Read the model definition and answer for the solid it produces. Units are mm, in the model's axes. Face numbers are marked on the shaded views. A direction names the side the tool comes from. Coordinates: 2 decimals unless noted, no trailing zeros. Write each loop counter-clockwise with the first axis right and the second up, starting at its lowest first coordinate (ties: lowest second). Pieces come first, ordered by that corner, then holes. Notation, with made-up numbers: (-25.5, 87.25) -> (-4.5, 87.25) arc R17 ccw to (-4.5, 113.25) -> close; hole circle Ø6 at (-38, 11.5). An arc over 180 degrees is marked (long way). Return JSON: item names as keys, results as strings.
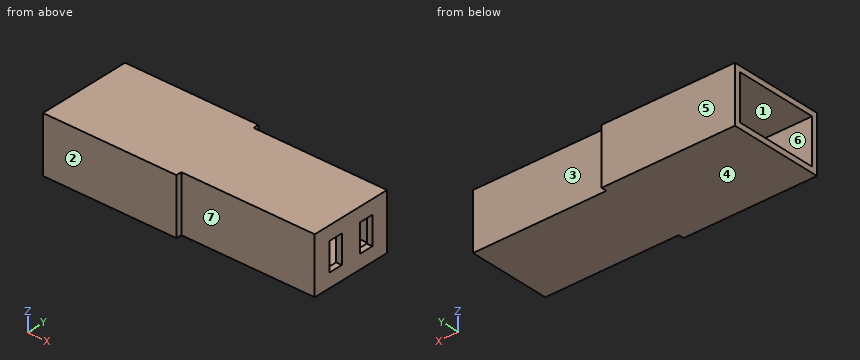
from build123d import *

# Parameters (mm, degrees)
F1_DEPTH = 4
F2_T     = -0.4
F3_W     = 1
F3_H     = 2
F4_DEPTH = 0.4


with BuildPart() as f1:
    # F0 (on Top) → F1 (new body)
    with BuildSketch(Plane.XY):
        Polygon((0, 3.35), (0, -3.35), (9.5, -3.35), (9.5, -2.95), (19, -2.95), (19, 2.95), (9.5, 2.95), (9.5, 3.35), align=None)
    extrude(amount=F1_DEPTH)

    # F2
    f2_openings = [f1.faces().sort_by_distance(p)[0] for p in [
        (0, 0, 2),
    ]]
    offset(amount=F2_T, openings=f2_openings, kind=Kind.INTERSECTION)

    # F3 (on face) → F4 (cut, through all)
    with BuildSketch(Plane.YZ.offset(19)):
        with Locations((-1.2436551969, 2)):
            Rectangle(F3_W, F3_H)
        with Locations((1.2563448031, 2)):
            Rectangle(F3_W, F3_H)
    extrude(amount=-F4_DEPTH, mode=Mode.SUBTRACT)


solid = f1.part
1. A tool of negligible diameter and unlimited length cuts with its end or side. For the marked faces 5, 6 and 7, from which of +Z, -Z, +X, -X, +Y, -Y can it reach the whole face along a straight path? Write none if from no direction.
Taken from the geometry:
{"face 5": "+Z, -Z, +X, -X, +Y", "face 6": "-X", "face 7": "+Z, -Z, +X, -Y"}
2. For a pull along Y with two mould halves and no side action, classify the marked faces 1, 2, 3 and 4 as +Y half, -Y half, draft (parallel to the pull), parting line (faces both ways), or undercut.
Taken from the geometry:
{"face 1": "undercut", "face 2": "-Y half", "face 3": "+Y half", "face 4": "draft"}
3. The part is cut by section C-C (z = 1.95). Determine the outline of the cut face in (x, y), then the cut area to 3 significant figures.
Taken from the geometry:
{"outline": "(0, -3.35) -> (9.5, -3.35) -> (9.5, -2.95) -> (19, -2.95) -> (19, -1.74) -> (18.6, -1.74) -> (18.6, -2.55) -> (9.1, -2.55) -> (9.1, -2.95) -> (0, -2.95) -> close; (0, 2.95) -> (9.1, 2.95) -> (9.1, 2.55) -> (18.6, 2.55) -> (18.6, 1.76) -> (19, 1.76) -> (19, 2.95) -> (9.5, 2.95) -> (9.5, 3.35) -> (0, 3.35) -> close; (18.6, -0.74) -> (19, -0.74) -> (19, 0.76) -> (18.6, 0.76) -> close", "area": "16.8 mm2"}
4. The part is cut by section A-A (x = 8.5). Determine the outline of the cut face in (y, z).
Taken from the geometry:
{"outline": "(-3.35, 0) -> (3.35, 0) -> (3.35, 4) -> (-3.35, 4) -> close; hole (-2.95, 0.4) -> (2.95, 0.4) -> (2.95, 3.6) -> (-2.95, 3.6) -> close"}
5. The part is cut by section D-D (y = 2.75). Determine the outline of the cut face in (x, z).
Taken from the geometry:
{"outline": "(0, 0) -> (19, 0) -> (19, 4) -> (0, 4) -> (0, 3.6) -> (9.1, 3.6) -> (9.1, 0.4) -> (0, 0.4) -> close"}
6. Flat-ended cylindrical pins translate along their axes: pin 1 Ø2 at (x, y) = (7.5, -1.5) entering from -Z; pin 2 Ø2 at (x, z) = (15.5, 3) entering from -Y. Find the tip coordinate at first contact, or state that the pin passes through.
Taken from the geometry:
{"pin 1": "stops at z = 0", "pin 2": "stops at y = -2.95"}
7. Consider L1, parallel to Y at x = 14.25, z = 0.5; L2, parallel to Y at x = 2, z = 2.8; L3, parallel to Z at x = 2, y = -1.5. Determine where each line is inside the solid, lowest interval first.
Taken from the geometry:
{"L1": "y = -2.95 to -2.55, 2.55 to 2.95", "L2": "y = -3.35 to -2.95, 2.95 to 3.35", "L3": "z = 0 to 0.4, 3.6 to 4"}
8. The part is cut by section B-B (y = 1.25). Determine the outline of the cut face in (x, z), then the cut area to 3 significant figures.
Taken from the geometry:
{"outline": "(0, 0) -> (19, 0) -> (19, 1) -> (18.6, 1) -> (18.6, 0.4) -> (0, 0.4) -> close; (0, 3.6) -> (18.6, 3.6) -> (18.6, 3) -> (19, 3) -> (19, 4) -> (0, 4) -> close", "area": "15.7 mm2"}
